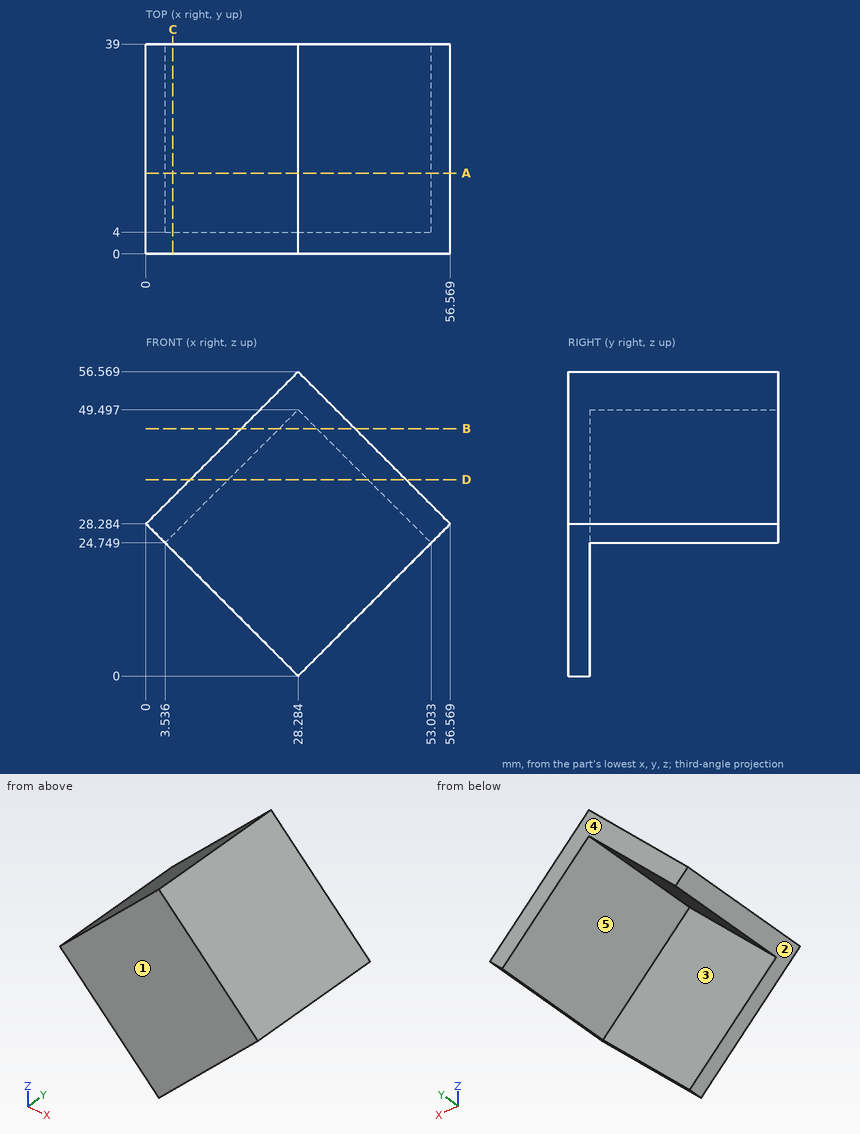
Design review of the part shown in the three views and the two pictorial views. Dimensions are in mm from the part's minimum x, y and z. A direction names the side the tool comes from. Round coordinates to 2 decimals unless told otherwise and drop trailing zeros. Loops run counter-clockwise (first coordinate to the right, second up) from the corner with the lowest first, then second, coordinate; pieces in that order, holes last.
(1) Clearance check with flat-ended pins moving along their axes: P1, Ø5, axis at x = 13, y = 6, coming from the -Z side (1 decimal); P2, Ø1, axis at x = 47.5, y = 8.5, coming from the -Z side; P3, Ø4, axis at x = 13, y = 4.5, coming from the +Z side (1 decimal). State where each tip first meets the part, or that it passes through.
Returned:
P1: stops at z = 13.8
P2: stops at z = 29.78
P3: stops at z = 43.3
(2) We need section C-C (x = 5). Give the boundary of the cut face in (y, z) (1 decimal).
Returned:
outline: (0, 23.3) - (4, 23.3) - (4, 26.2) - (39, 26.2) - (39, 33.3) - (0, 33.3) - close
(3) Wall thickness on line 1 along Y through (x, z) = (30, 32.5); line 2 along X through (y, z) = (25.5, 27.5) (1 decimal); line 3 along Z through (x, y) = (22, 15) (1 decimal): over which ranges is each line inside the solid? List them lowest first.
Returned:
line 1: y = 0 to 4
line 2: x = 0.8 to 6.3, 50.3 to 55.8
line 3: z = 43.2 to 50.3
(4) We need section A-A (y = 15). Give the boundary of the cut face in (x, z) (1 decimal), plus the area to 3 significant figures.
Returned:
outline: (0, 28.3) - (3.5, 24.7) - (28.3, 49.5) - (53, 24.7) - (56.6, 28.3) - (28.3, 56.6) - close
area: 375 mm2
(5) We need section B-B (z = 46). Give the boundary of the cut face in (x, y) (1 decimal).
Returned:
outline: (17.7, 0) - (38.9, 0) - (38.9, 39) - (31.8, 39) - (31.8, 4) - (24.8, 4) - (24.8, 39) - (17.7, 39) - close
(6) Mouldability with a two-part tool opening along X and no side actions: class the marked faces 1, 2 and 3 as released by +X, released by -X, zero draft, split by the parting line, or undercut.
Returned:
face 1: zero draft
face 2: released by -X
face 3: undercut
(7) Tool access review of the marked faces 4 and 5: name each direction out of +Z, -Z, +X, -X, +Y, -Y from which nothing blocks a thin tool from reaching the whole face with its end or side.
Returned:
face 4: +Z, -Z, +X, -X, +Y
face 5: -Z, +Y
(8) We need section D-D (z = 36.5). Give the boundary of the cut face in (x, y) (1 decimal).
Returned:
outline: (8.2, 0) - (48.4, 0) - (48.4, 39) - (41.3, 39) - (41.3, 4) - (15.3, 4) - (15.3, 39) - (8.2, 39) - close
